Here's the drawing with two shaded views (mm, measured from the low corner). I have some questions. A direction names the side the tool comes from. Coordinates: 2 decimals unless noted, no trailing zeros. Loops run counter-clockwise (first coordinate to the right, second up) from the corner with the lowest first, then second, coordinate; pieces in that order, holes last.
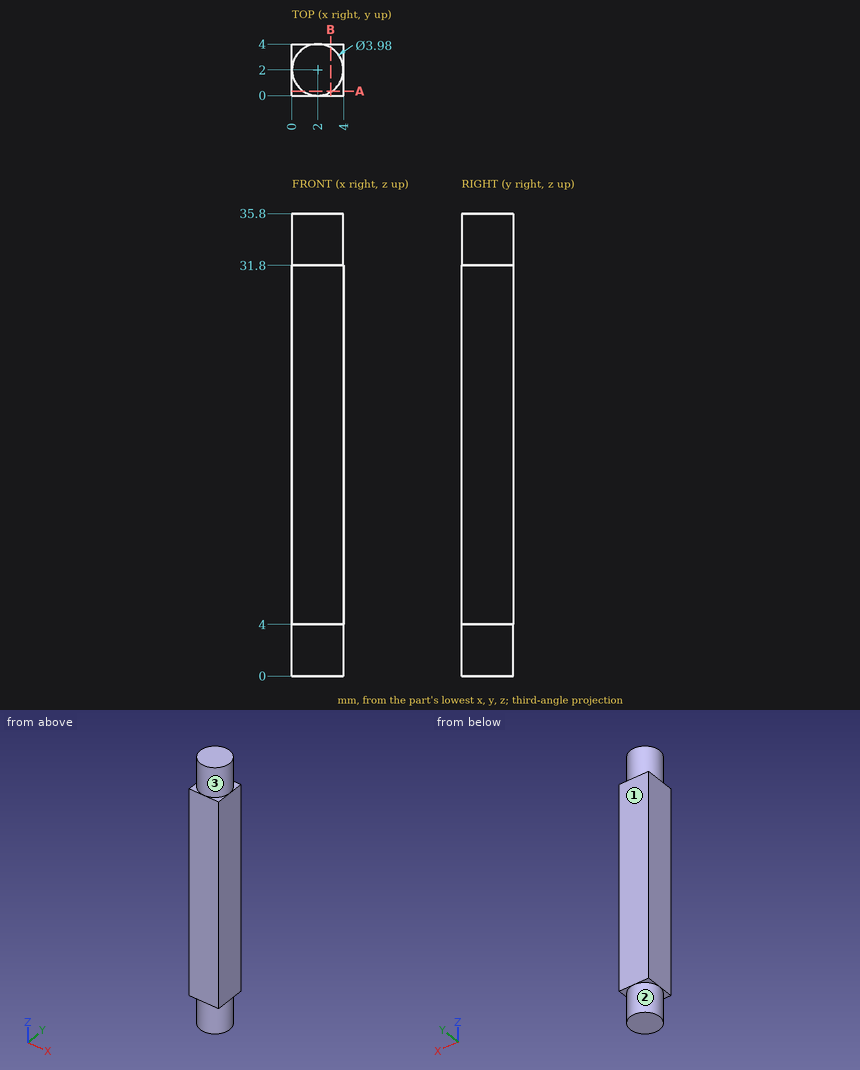
(1) If I drill on probe 1 along X at (y, z) = (0.3, 2); probe 2 along Y at (x, z) = (0.45, 33.5), over which ranges is the centre line in solid material (lowest first)?
Check values:
probe 1: x = 0.97 to 3.03
probe 2: y = 0.75 to 3.25
(2) I'm going to push a flat-ended pin straight in: pin 1 (2 mm diameter, centred on y = 2.5, z = 8.5, fed in from -X). Where does the tip first touch, or does it pass through?
Check values:
pin 1: stops at x = 0
(3) I want a section at B-B on x = 3. Write out the boundary of the cut face in (y, z).
Check values:
outline: (0, 4) - (0.28, 4) - (0.28, 0) - (3.72, 0) - (3.72, 4) - (4, 4) - (4, 31.8) - (3.72, 31.8) - (3.72, 35.8) - (0.28, 35.8) - (0.28, 31.8) - (0, 31.8) - close
(4) Which directions (+Z, -Z, +X, -X, +Y, -Y) give clear straight access to the entire face, cutting with the end or side of a thin tool? Please do the marked faces 1, 2 and 3.
Check values:
face 1: +Z, -Z, +X, -X, +Y
face 2: -Z
face 3: +Z
(5) I want a section at A-A on y = 0.35. Write out the boundary of the cut face in (x, z), then the cut area to 3 significant figures.
Check values:
outline: (0, 4) - (0.89, 4) - (0.89, 0) - (3.11, 0) - (3.11, 4) - (4, 4) - (4, 31.8) - (3.11, 31.8) - (3.11, 35.8) - (0.89, 35.8) - (0.89, 31.8) - (0, 31.8) - close
area: 129 mm2
